Check sheet for the drawn part. Datum: minimum x, y, z corner. Units: mm. Round coordinates to 2 decimals unless told otherwise and drop trailing zeros. Write each loop counter-clockwise with the first axis right and the second up, starting at its lowest first coordinate (ties: lowest second). Pieces come first, ordered by that corner, then holes. Notation, with made-up numbers: (65.25, 47.5) - (124.25, 47.5) arc R26 cw to (124.25, 66.5) - close; hole circle Ø1 at (30, 15). An arc over 180 degrees is marked (long way). Answer as a JSON object with one key per item and string values. Group by question number.
1) Thickness scan on line 1 (Y direction, x = 10, z = 11.75); line 2 (Y direction, x = 10, z = 5.5); line 3 (Y direction, x = 16.75, z = 23.5). Record the ranges inside material, lowest first.
2) Section check A-A (z = 18.5). Enter the section's corners in (x, y), then the cut area to 3 significant figures.
3) Go/stop test with flat-tipped pins: pin 1 Ø12 at (x, z) = (17, 16.5) entering from -Y; pin 2 Ø5 at (x, z) = (16, 21) entering from +Y; pin 3 Ø1.5 at (x, z) = (15.5, 17.5) entering from +Y. Record where each tip stops, or that it passes through.
4) Mould release check, pull along X, two halves, no side actions. Record for the marked faces 1, 2 and 3: +X half, -X half, draft (parallel to the pull), parting line (faces both ways), or undercut.
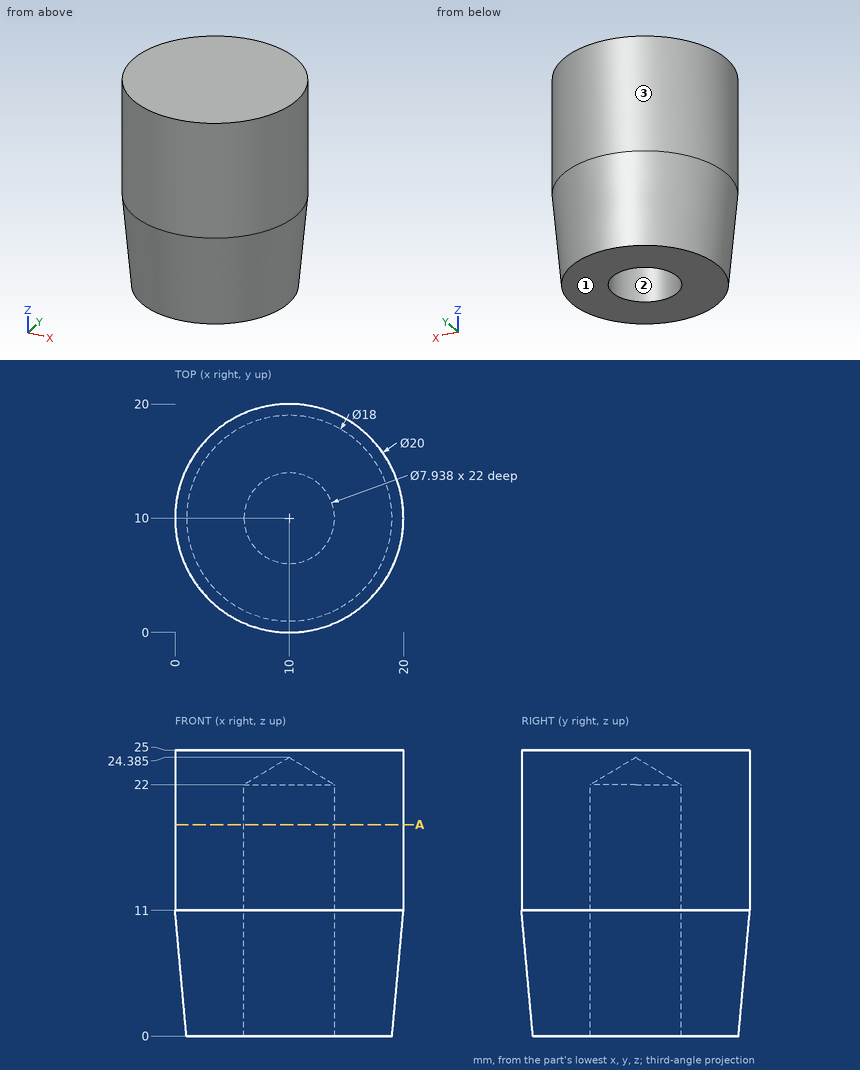
Returned:
{
 "1": {"line 1": "0 to 6.03, 13.97 to 20", "line 2": "0.5 to 6.03, 13.97 to 19.5", "line 3": "2.62 to 17.38"},
 "2": {"outline": "circle Ø20 at (10, 10); hole circle Ø7.94 at (10, 10)", "area": "265 mm2"},
 "3": {"pin 1": "y = 0.05", "pin 2": "y = 19.37", "pin 3": "y = 18.8"},
 "4": {"face 1": "draft", "face 2": "undercut", "face 3": "parting line"}
}
